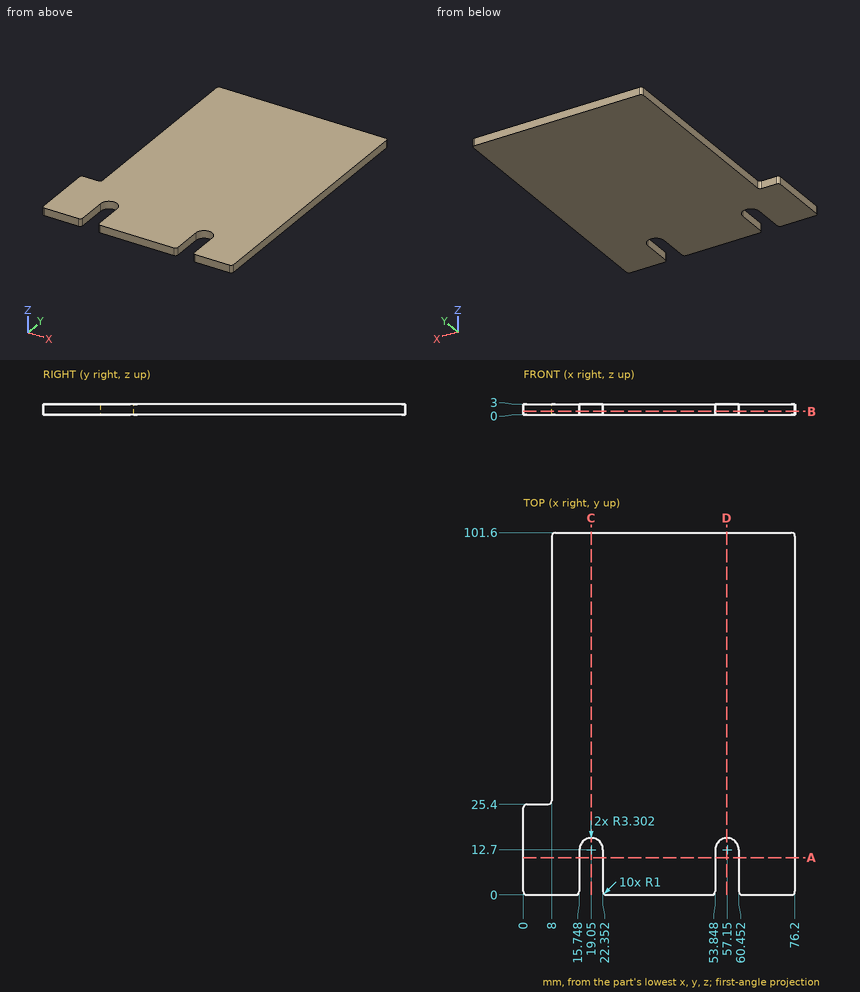
For this review, use the dimensioned drawing (mm, ordinates from the lowest corner) and the shaded views. Round coordinates to 2 decimals unless told otherwise and drop trailing zeros. Write each loop counter-clockwise with the first axis right and the second up, starting at its lowest first coordinate (ties: lowest second). Pieces come first, ordered by that corner, then holes. Notation, with made-up numbers: M 56,-4 L 87,-4 A27 cw 87,33 Z; hole C 16,36 d8. An arc over 180 degrees is marked long. Write item = value, one per line. Start each with the question number.
(1) We need section C-C (x = 19.05). Give the boundary of the cut face in (y, z), then the cut area to 3 significant figures.
(2) We need section A-A (y = 10.5). Give the boundary of the cut face in (x, z), then the cut area to 3 significant figures.
(3) For line 1 along X through (y, z) = (15, 2.8); line 2 along X through (y, z) = (37.5, 2.5); line 3 along Y through (x, z) = (5, 1), list the stretches that pass through material, from the lowest coordinate up.
(4) We need section B-B (z = 0.95). Give the boundary of the cut face in (x, y).
Results found:
q1.outline = M 16,0 L 101.6,0 L 101.6,3 L 16,3 Z
q1.area = 257 mm²
q2.outline = M 0,0 L 15.75,0 L 15.75,3 L 0,3 Z; M 22.35,0 L 53.85,0 L 53.85,3 L 22.35,3 Z; M 60.45,0 L 76.2,0 L 76.2,3 L 60.45,3 Z
q2.area = 189 mm²
q3.line_1 = 0 to 16.68, 21.42 to 54.78, 59.52 to 76.2
q3.line_2 = 8 to 76.2
q3.line_3 = 0 to 25.4
q4.outline = M 0,1 A1 ccw 1,0 L 14.75,0 A1 ccw 15.75,1 L 15.75,12.7 A3.3 cw 22.35,12.7 L 22.35,1 A1 ccw 23.35,0 L 52.85,0 A1 ccw 53.85,1 L 53.85,12.7 A3.3 cw 60.45,12.7 L 60.45,1 A1 ccw 61.45,0 L 75.2,0 A1 ccw 76.2,1 L 76.2,100.6 A1 ccw 75.2,101.6 L 9,101.6 A1 ccw 8,100.6 L 8,26.4 A1 cw 7,25.4 L 1,25.4 A1 ccw 0,24.4 Z
